The model under review builds one solid part; all positions refer to its coordinate system, in mm. Face numbers are marked on the shaded views. Coordinates: 2 decimals unless noted, no trailing zeros. Loops run counter-clockwise (first coordinate to the right, second up) from the corner with the lowest first, then second, coordinate; pieces in that order, holes last. Notation, with made-up numbers: M 78.25,7 L 108.25,7 A24 ccw 108.25,39 Z; hole C 15.25,75.5 d9. An arc over 180 degrees is marked long. Use one line per item in the form item = value.
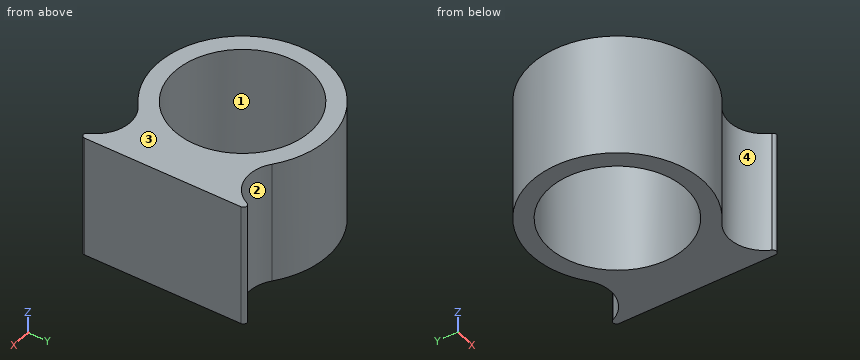
```python
from build123d import *

# Parameters (mm, degrees)
F0_R     = 9.75
F1_DEPTH = 17.5
F2_R     = 5
F3_R     = 0.5


with BuildPart() as f1:
    # F0 (on Top) → F1 (new body)
    with BuildSketch(Plane.XY):
        with BuildLine():
            Line((16.25, 13.347993), (11.627468, 3.85545))
            ThreePointArc((11.627468, 3.85545), (-12.25, 0), (11.627468, -3.85545))
            Line((11.627468, -3.85545), (16.25, -13.347993))
            Line((16.25, -13.347993), (16.25, 13.347993))
        make_face()
        Circle(F0_R, mode=Mode.SUBTRACT)
    extrude(amount=F1_DEPTH)

    # F2
    f2_edges = [f1.edges().sort_by_distance(p)[0] for p in [
        (11.627468, -3.85545, 8.75),
        (11.627468, 3.85545, 8.75),
    ]]
    fillet(f2_edges, radius=F2_R)

    # F3
    f3_edges = [f1.edges().sort_by_distance(p)[0] for p in [
        (16.25, 13.347993, 8.75),
        (16.25, -13.347993, 8.75),
    ]]
    fillet(f3_edges, radius=F3_R)


solid = f1.part
```
1. Add section C-C (z = 3.25). State the section outline as (x, y) points, then the cut area to 3 significant figures.
Response values:
outline = M 7.64,-9.58 A5 cw 15.25,-11.3 L 15.3,-11.4 A0.5 ccw 16.25,-11.18 L 16.25,11.18 A0.5 ccw 15.3,11.4 L 15.25,11.3 A5 cw 7.64,9.58 A12.25 ccw long Z; hole C 0,0 d19.5
area = 273 mm^2
2. Add section D-D (x = 14). State the section outline as (y, z) points, then the cut area to 3 significant figures.
Response values:
outline = M -9.68,0 L 9.68,0 L 9.68,17.5 L -9.68,17.5 Z
area = 339 mm^2
3. Add section B-B (y = 0). State the section outline as (x, z) points.
Response values:
outline = M -12.25,0 L -9.75,0 L -9.75,17.5 L -12.25,17.5 Z; M 9.75,0 L 16.25,0 L 16.25,17.5 L 9.75,17.5 Z
4. Add section A-A (x = 0). State the section outline as (y, z) points, then the cut area to 3 significant figures.
Response values:
outline = M -12.25,0 L -9.75,0 L -9.75,17.5 L -12.25,17.5 Z; M 9.75,0 L 12.25,0 L 12.25,17.5 L 9.75,17.5 Z
area = 87.5 mm^2
5. The part is to be moulded in two halves that separate along Y. For the marked faces 1, 2, 3 and 4, say which applies: pulls with the +Y half, pulls with the -Y half, needs draft (parallel to the pull), parting line crosses it, or undercut.
Response values:
face_1 = undercut
face_2 = pulls with the +Y half
face_3 = needs draft
face_4 = pulls with the -Y half
6. Insertion check: P1, Ø2, axis at x = -9, y = -2, coming from the +Z side; P2, Ø1, axis at x = -3.5, z = 11, coming from the +Y side; P3, Ø4, axis at y = -3.5, z = 5, coming from the -X side; P4, Ø10, axis at x = 9, z = 14.5, coming from the -Y side. Each pin has a flat end and moves straight along its axis. Give the tip position at first contact, or say it passes through.
Response values:
P1 = 17.5
P2 = 11.88
P3 = -12.16
P4 = -11.58
7. Wall thickness on line 1 along Y through (x, z) = (0, 4); line 2 along Y through (x, z) = (10.5, 15.75); line 3 along X through (y, z) = (3.75, 4.75): over which ranges is each line inside the solid? List them lowest first. Write a range as from..to.
Response values:
line_1 = -12.25..-9.75, 9.75..12.25
line_2 = -8.49..8.49
line_3 = -11.66..-9, 9..16.25
